```python
from build123d import *

# Parameters (mm, degrees)
SKETCH1_W                                        = 50
SKETCH1_H                                        = 110
BOSS_EXTRUDE1_DEPTH                              = 10
CSK_FOR_1_4_FLAT_HEAD_MACHINE_SCREW1_D           = 6.5278
CSK_FOR_1_4_FLAT_HEAD_MACHINE_SCREW1_CSINK_D     = 12.8778
CSK_FOR_1_4_FLAT_HEAD_MACHINE_SCREW1_CSINK_ANGLE = 82
FILLET1_R                                        = 2


with BuildPart() as part:
    # Sketch1 → Boss-Extrude1 (new body)
    with BuildSketch(Plane.XY):
        with Locations((0.542522126, -0.271261063)):
            Rectangle(SKETCH1_W, SKETCH1_H)
        Polygon((0.542522126, 16.44340804), (6.992522126, 16.44340804), (6.992522126, -15.50659196), (0.542522126, -15.50659196), (-5.907477874, -15.50659196), (-5.907477874, 16.44340804), align=None, mode=Mode.SUBTRACT)
    extrude(amount=BOSS_EXTRUDE1_DEPTH)

    # CSK for 1/4 Flat Head Machine Screw1 (through all)
    with Locations(Plane.XY.offset(10)):
        with Locations((0.542522126, -35.581261063), (0.542522126, 35.038738937)):
            CounterSinkHole(CSK_FOR_1_4_FLAT_HEAD_MACHINE_SCREW1_D / 2, CSK_FOR_1_4_FLAT_HEAD_MACHINE_SCREW1_CSINK_D / 2, counter_sink_angle=CSK_FOR_1_4_FLAT_HEAD_MACHINE_SCREW1_CSINK_ANGLE)

    # Fillet1
    fillet1_edges = [part.edges().sort_by_distance(p)[0] for p in [
        (-24.457477874, 54.728738937, 5),
        (25.542522126, 54.728738937, 5),
        (25.542522126, -55.271261063, 5),
        (-24.457477874, -55.271261063, 5),
    ]]
    fillet(fillet1_edges, radius=FILLET1_R)


solid = part.part
```
Can you work these out from the model? Positions are in its coordinate system, mm. A direction names the side the tool comes from. Coordinates: 2 decimals unless noted, no trailing zeros. Loops run counter-clockwise (first coordinate to the right, second up) from the corner with the lowest first, then second, coordinate; pieces in that order, holes last.
Item 1: Please list where these lines run through material, in increasing order: L1, parallel to Y at x = -3, z = 1.5; L2, parallel to X at y = 6, z = 6.25; L3, parallel to Y at x = 1, z = 3.
Answers below:
L1: y = -55.27 to -15.51, 16.44 to 54.73
L2: x = -24.46 to -5.91, 6.99 to 25.54
L3: y = -55.27 to -38.81, -32.35 to -15.51, 16.44 to 31.81, 38.27 to 54.73
Item 2: Which directions (+Z, -Z, +X, -X, +Y, -Y) give clear straight access to the entire face, cutting with the end or side of a thin tool? Please do faces 4 (the face through (6.993, 1, 5)), 5 (the face through (-1.295, 37.921, 6.525)).
Answers below:
face 4: +Z, -Z
face 5: +Z
Item 3: Suppose I cut it at B-B (z = 9). Please give me the cut outline in (x, y).
Answers below:
outline: (-24.46, -53.27) arc R2 ccw to (-22.46, -55.27) - (23.54, -55.27) arc R2 ccw to (25.54, -53.27) - (25.54, 52.73) arc R2 ccw to (23.54, 54.73) - (-22.46, 54.73) arc R2 ccw to (-24.46, 52.73) - close; hole (-5.91, -15.51) - (6.99, -15.51) - (6.99, 16.44) - (-5.91, 16.44) - close; hole circle Ø11.14 at (0.54, -35.58); hole circle Ø11.14 at (0.54, 35.04)
Item 4: If we mould it in two halves opening along Y, with no side actions, what happens to faces 1 (the face through (-24, 54, 5)), 2 (the face through (-1.295, -32.699, 6.525)), 3 (the face through (0, -55.271, 5))? For each: released by +Y, released by -Y, zero draft, split by the parting line, or undercut.
Answers below:
face 1: released by +Y
face 2: undercut
face 3: released by -Y
Item 5: Suppose I cut it at C-C (z = 4). Please give me the cut outline in (x, y), then the cut area to 3 significant figures.
Answers below:
outline: (-24.46, -53.27) arc R2 ccw to (-22.46, -55.27) - (23.54, -55.27) arc R2 ccw to (25.54, -53.27) - (25.54, 52.73) arc R2 ccw to (23.54, 54.73) - (-22.46, 54.73) arc R2 ccw to (-24.46, 52.73) - close; hole (-5.91, -15.51) - (6.99, -15.51) - (6.99, 16.44) - (-5.91, 16.44) - close; hole circle Ø6.53 at (0.54, -35.58); hole circle Ø6.53 at (0.54, 35.04)
area: 5,020 mm2
Item 6: I'm going to push a flat-ended pin straight in: pin 1 (7.5 mm diameter, centred on x = 0.54, y = -35.58, fed in from +Z). Where does the tip first touch, or does it pass through?
Answers below:
pin 1: stops at z = 6.91
Item 7: Suppose I cut it at A-A (y = -1). Please give me the cut outline in (x, z).
Answers below:
outline: (-24.46, 0) - (-5.91, 0) - (-5.91, 10) - (-24.46, 10) - close; (6.99, 0) - (25.54, 0) - (25.54, 10) - (6.99, 10) - close
